from build123d import *

# Parameters (mm, degrees)
SKETCH_1_R                = 45
SKETCH_1_R_2              = 36
EXTRUDE_1_DEPTH           = 19
EXTRUDE_START             = -10
SKETCH_1_3_W              = 130
SKETCH_1_3_H              = 130
SKETCH_1_3_R              = 2.5
SKETCH_1_3_R_2            = 45
SKETCH_1_3_R_3            = 36
EXTRUDE_2_DEPTH           = 10
SKETCH_1_4_W              = 130
SKETCH_1_4_H              = 130
SKETCH_1_4_R              = 2.5
SKETCH_1_4_R_2            = 45
EXTRUDE_3_DEPTH           = 7.7
HOLE_WIZARD_1_D           = 5.5
HOLE_WIZARD_1_CBORE_D     = 10
HOLE_WIZARD_1_CBORE_DEPTH = 5.7
CHAMFER_1_SIZE            = 10


with BuildPart() as part:
    # Sketch 1 → Extrude 1 (new body)
    with BuildSketch(Plane.XY):
        Circle(SKETCH_1_R)
        Circle(SKETCH_1_R_2, mode=Mode.SUBTRACT)
    extrude(amount=EXTRUDE_1_DEPTH)

    # Sketch 1_3 → Extrude 2 (add)
    # profile 1 of 3: a face of its own
    with BuildSketch(Plane.XY.offset(EXTRUDE_START)):
        Rectangle(SKETCH_1_3_W, SKETCH_1_3_H)
        with Locations((-42.426406871, -42.426406871)):
            Circle(SKETCH_1_3_R, mode=Mode.SUBTRACT)
        with Locations((42.426406871, -42.426406871)):
            Circle(SKETCH_1_3_R, mode=Mode.SUBTRACT)
        with Locations((42.426406871, 42.426406871)):
            Circle(SKETCH_1_3_R, mode=Mode.SUBTRACT)
        with Locations((-42.426406871, 42.426406871)):
            Circle(SKETCH_1_3_R, mode=Mode.SUBTRACT)
        Circle(SKETCH_1_3_R_2, mode=Mode.SUBTRACT)
    # profile 2 of 3: a face of its own
    with BuildSketch(Plane.XY.offset(EXTRUDE_START)):
        Circle(SKETCH_1_3_R_2)
        Circle(SKETCH_1_3_R_3, mode=Mode.SUBTRACT)
    # profile 3 of 3: a face of its own
    with BuildSketch(Plane.XY.offset(EXTRUDE_START)):
        Circle(SKETCH_1_3_R_3)
    extrude(amount=EXTRUDE_2_DEPTH)

    # Sketch 1_4 → Extrude 3 (add)
    with BuildSketch(Plane.XY):
        Rectangle(SKETCH_1_4_W, SKETCH_1_4_H)
        with Locations((-42.426406871, -42.426406871)):
            Circle(SKETCH_1_4_R, mode=Mode.SUBTRACT)
        with Locations((42.426406871, -42.426406871)):
            Circle(SKETCH_1_4_R, mode=Mode.SUBTRACT)
        with Locations((42.426406871, 42.426406871)):
            Circle(SKETCH_1_4_R, mode=Mode.SUBTRACT)
        with Locations((-42.426406871, 42.426406871)):
            Circle(SKETCH_1_4_R, mode=Mode.SUBTRACT)
        Circle(SKETCH_1_4_R_2, mode=Mode.SUBTRACT)
    extrude(amount=EXTRUDE_3_DEPTH)

    # Hole Wizard 1 (through all)
    with Locations(Plane(origin=(0, 0, -10), x_dir=(-1, 0, 0), z_dir=(0, 0, -1))):
        with Locations((42.426406871, 42.426406871), (-42.426406871, 42.426406871), (42.426406871, -42.426406871), (-42.426406871, -42.426406871)):
            CounterBoreHole(HOLE_WIZARD_1_D / 2, HOLE_WIZARD_1_CBORE_D / 2, HOLE_WIZARD_1_CBORE_DEPTH)

    # Chamfer 1
    chamfer_1_edges = [part.edges().sort_by_distance(p)[0] for p in [
        (-65, -65, -1.15),
        (-65, 65, -1.15),
        (65, 65, -1.15),
        (65, -65, -1.15),
    ]]
    chamfer(chamfer_1_edges, length=CHAMFER_1_SIZE)


solid = part.part
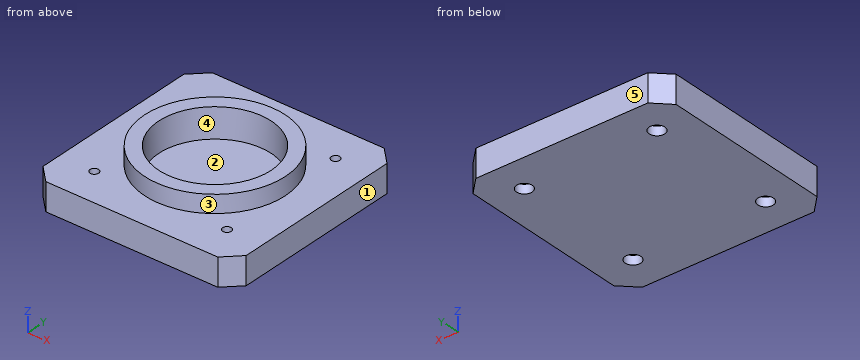
CAD build for the part. Positions are in the model's coordinates, mm. Face numbers are marked on the shaded views. A direction names the side the tool comes from. Give positions to 0.01 mm unless a question says otherwise; leave off trailing zeros. Loops run counter-clockwise (first coordinate to the right, second up) from the corner with the lowest first, then second, coordinate; pieces in that order, holes last. Notation, with made-up numbers: M 50.5,62.5 L 102.5,62.5 A9 cw 102.5,71.5 Z; hole C 89,28 d1. An arc over 180 degrees is marked long. Write each question's results on one line, items separated by ' | '.
Q1. Band-saw the part on D-D on z = 17.5. Write the cut outline in (x, y), and give its area (3 significant figures).
Geometry check:
outline: C 0,0 d90; hole C 0,0 d72 | area: 2,290 mm²
Q2. Which spindle directions (+Z, -Z, +X, -X, +Y, -Y) get a long thin tool onto all of the face, cutting with end or side? Do the marked faces 4 and 5. Say none if no direction does.
Geometry check:
face 4: +Z | face 5: +Z, -Z, +X, -X, +Y
Q3. Band-saw the part on C-C on z = -8. Write the cut outline in (x, y), and give its area (3 significant figures).
Geometry check:
outline: M -65,-55 L -55,-65 L 55,-65 L 65,-55 L 65,55 L 55,65 L -55,65 L -65,55 Z; hole C -42.43,-42.43 d10; hole C -42.43,42.43 d10; hole C 42.43,-42.43 d10; hole C 42.43,42.43 d10 | area: 16,400 mm²
Q4. Flat gauge pins, fed straight in: P1, Ø9, axis at x = 42.43, y = -42.43, coming from the +Z side; P2, Ø5, axis at x = -44.5, y = 42.5, coming from the -Z side; P3, Ø5, axis at y = 39, z = 15, coming from the -X side. Where does each tip first touch, or does it go through?
Geometry check:
P1: stops at z = 7.7 | P2: stops at z = -4.3 | P3: stops at x = -26.32
Q5. Mould opens along Y. For the marked faces 1, 2 and 3 say: pulls with the +Y half, pulls with the -Y half, needs draft (parallel to the pull), parting line crosses it, or undercut.
Geometry check:
face 1: needs draft | face 2: undercut | face 3: parting line crosses it
Q6. Band-saw the part on A-A on y = 0. Write the cut outline in (x, z).
Geometry check:
outline: M -65,-10 L 65,-10 L 65,7.7 L 45,7.7 L 45,19 L 36,19 L 36,0 L -36,0 L -36,19 L -45,19 L -45,7.7 L -65,7.7 Z
Q7. Probe probe 1 along X at (y, z) = (-42.5, -4.25); probe 2 along Y at (x, z) = (0, 5). List the from-to ranges inside material, lowest first.
Geometry check:
probe 1: x = -65 to -45.18, -39.68 to 39.68, 45.18 to 65 | probe 2: y = -65 to -36, 36 to 65
